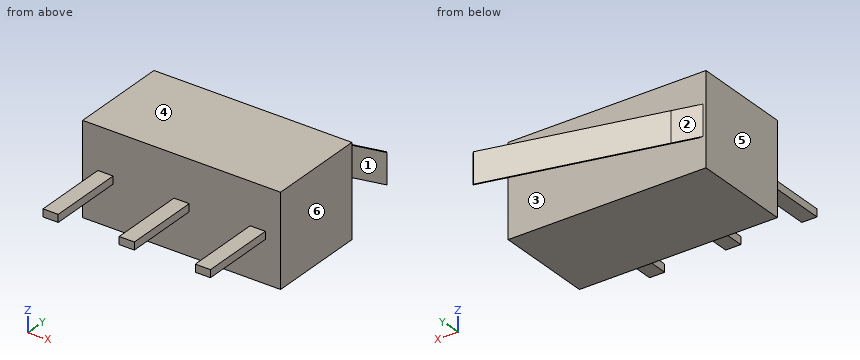
```python
from build123d import *

# Parameters (mm, degrees)
ESQUISSE1_W        = 13
ESQUISSE1_H        = 6
BOSS_EXTRU_1_DEPTH = 6.5
ESQUISSE2_W        = 1
ESQUISSE2_H        = 0.5
BOSS_EXTRU_2_DEPTH = 5
BOSS_EXTRU_3_DEPTH = 1


with BuildPart() as part:
    # Esquisse1 → Boss.-Extru.1 (new body)
    with BuildSketch(Plane(origin=(0, 0, 0), x_dir=(1, 0, 0), z_dir=(0, 1, 0))):
        Rectangle(ESQUISSE1_W, ESQUISSE1_H)
    extrude(amount=BOSS_EXTRU_1_DEPTH)

    # Esquisse2 → Boss.-Extru.2 (add)
    with BuildSketch(Plane.XZ):
        with Locations((-5, 0)):
            Rectangle(ESQUISSE2_W, ESQUISSE2_H)
        Rectangle(ESQUISSE2_W, ESQUISSE2_H)
        with Locations((5, 0)):
            Rectangle(ESQUISSE2_W, ESQUISSE2_H)
    extrude(amount=BOSS_EXTRU_2_DEPTH)

    # Esquisse3 → Boss.-Extru.3 (add, symmetric)
    with BuildSketch(Plane.XY):
        Polygon((-6.00813505, 6.5), (6.640975591, 9.5), (6.555428051, 9.551784345), (-4.520695815, 6.924850916), (-6.3, 6.5), align=None)
    extrude(amount=BOSS_EXTRU_3_DEPTH, both=True)


solid = part.part
```
Geometry: final body of the model. Coordinates: model frame, mm. Face numbers are marked on the shaded views. A direction names the side the tool comes from. Round coordinates to 2 decimals unless told otherwise and drop trailing zeros. Order: outer loops, then holes, each group sorted by start corner. A loop starts at its lowest first (then second) coordinate and runs counter-clockwise, first axis right, second up. Notation, with made-up numbers: M 50.5,9 L 75.5,9 A8 cw 75.5,22 Z; hole C 27,-0.75 d1. An arc over 180 degrees is marked long. One line per item, written item: value.
(1) Cut plane B-B (z = 0.55). Return the cut outline in (x, y).
Result sheet:
outline: M -6.5,0 L 6.5,0 L 6.5,6.5 L -6.01,6.5 L 6.64,9.5 L 6.56,9.55 L -4.52,6.92 L -6.3,6.5 L -6.5,6.5 Z
(2) Cut plane D-D (y = 7.5). Return the cut outline in (x, z).
Result sheet:
outline: M -2.1,-1 L -1.79,-1 L -1.79,1 L -2.1,1 Z
(3) Pull-direction query (Y, two-part tool) for the marked faces 1, 2, 3 and 4; classes: pulls with the +Y half, pulls with the -Y half, needs draft (parallel to the pull), parting line crosses it, or undercut.
Result sheet:
face 1: undercut
face 2: pulls with the +Y half
face 3: undercut
face 4: needs draft
(4) Pin query (flat end, axial travel): P1, Ø1.1, axis at x = 0, y = -3.5, coming from the -Z side; P2, Ø1.8, axis at x = -2, z = 0, coming from the +Y side; P3, Ø1.5, axis at x = 2, y = 8, coming from the +Z side; P4, Ø3, axis at x = 0, z = -1, coming from the -Y side. Return the tip coordinate at first contact, or that it passes through.
Result sheet:
P1: z = -0.25
P2: y = 7.74
P3: z = 1
P4: y = -5
(5) Cut plane A-A (y = -0.25). Return the cut outline in (x, z), and give its area (3 significant figures).
Result sheet:
outline: M -5.5,-0.25 L -4.5,-0.25 L -4.5,0.25 L -5.5,0.25 Z; M -0.5,-0.25 L 0.5,-0.25 L 0.5,0.25 L -0.5,0.25 Z; M 4.5,-0.25 L 5.5,-0.25 L 5.5,0.25 L 4.5,0.25 Z
area: 1.50 mm2
(6) Line query: probe 1 along Y at (x, z) = (-4, -1.75); probe 2 along X at (y, z) = (4.25, -0.75); probe 3 along Z at (x, y) = (-0.25, -0.5). Output: solid intervals per line, ascending. Write a range as [from, to].
Result sheet:
probe 1: [0, 6.5]
probe 2: [-6.5, 6.5]
probe 3: [-0.25, 0.25]
(7) Cut plane C-C (x = -3.5). Return the cut outline in (y, z).
Result sheet:
outline: M 0,-3 L 6.5,-3 L 6.5,3 L 0,3 Z; M 7.09,-1 L 7.17,-1 L 7.17,1 L 7.09,1 Z
(8) Reachability of the marked faces 5 and 6 from +Z, -Z, +X, -X, +Y, -Y: full face, straight path, thin tool, end or side. Return the list, or none.
Result sheet:
face 5: +Z, -Z, -X, +Y, -Y
face 6: +Z, -Z, +X, -Y
